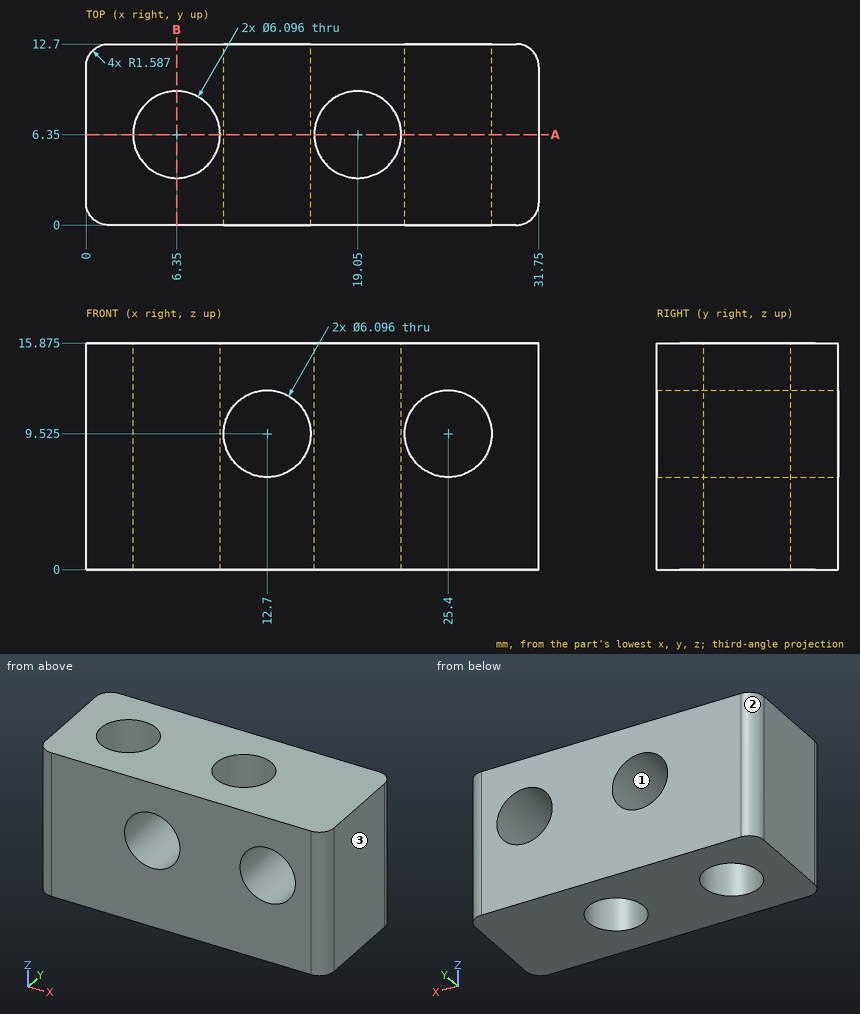
The drawing under review shows one solid part. Ordinate dimensions are in mm from its lowest x, y, z. Give positions to 0.01 mm unless a question says otherwise; leave off trailing zeros. Order: outer loops, then holes, each group sorted by start corner. A loop starts at its lowest first (then second) coordinate and runs counter-clockwise, first axis right, second up. Notation, with made-up numbers: M 2.25,12 L 26.25,12 A17 ccw 26.25,34 Z; hole C 45,66 d11. An arc over 180 degrees is marked long. Answer in a Markdown table with one row per item. Add a question column.
1. Add section A-A on y = 6.35. Count the separate pieces of the cut face and the enclosed holes in it, plus the area to 3 significant figures.
2. Add section B-B on x = 6.35. State the section outline as (y, z) points (1 decimal).
3. Mouldability with a two-part tool opening along X and no side actions: class the marked faces 1, 2 and 3 as released by +X, released by -X, zero draft, split by the parting line, or undercut.
4. To check wall thickness, follow line 1 along Y through (x, z) = (19.05, 7); line 2 along Z through (x, y) = (12.7, 9) (1 decimal); line 3 along X through (y, z) = (7.75, 14). State the ranges of each line that lie inside material, in increasing order.
The answers:
| question | item | result |
|---|---|---|
| 1 | separate pieces | 3 |
| 1 | enclosed holes | 2 |
| 1 | area | 252 mm2 |
| 2 | outline | M 0,0 L 3.3,0 L 3.3,15.9 L 0,15.9 Z; M 9.4,0 L 12.7,0 L 12.7,15.9 L 9.4,15.9 Z |
| 3 | face 1 | undercut |
| 3 | face 2 | released by -X |
| 3 | face 3 | released by +X |
| 4 | line 1 | 0 to 3.3, 9.4 to 12.7 |
| 4 | line 2 | 0 to 6.5, 12.6 to 15.9 |
| 4 | line 3 | 0 to 3.64, 9.06 to 16.34, 21.76 to 31.75 |
